Verification items for this drawing (mm, ordinates from the low corner). A direction names the side the tool comes from. Give positions to 0.01 mm unless a question says otherwise; leave off trailing zeros. Loops run counter-clockwise (first coordinate to the right, second up) from the corner with the lowest first, then second, coordinate; pieces in that order, holes last. Notation, with made-up numbers: M 3,38.25 L 58,38.25 A25 cw 58,74.25 Z; hole C 2,70 d1. An arc over 180 degrees is marked long. Use one line per item in the form item = value.
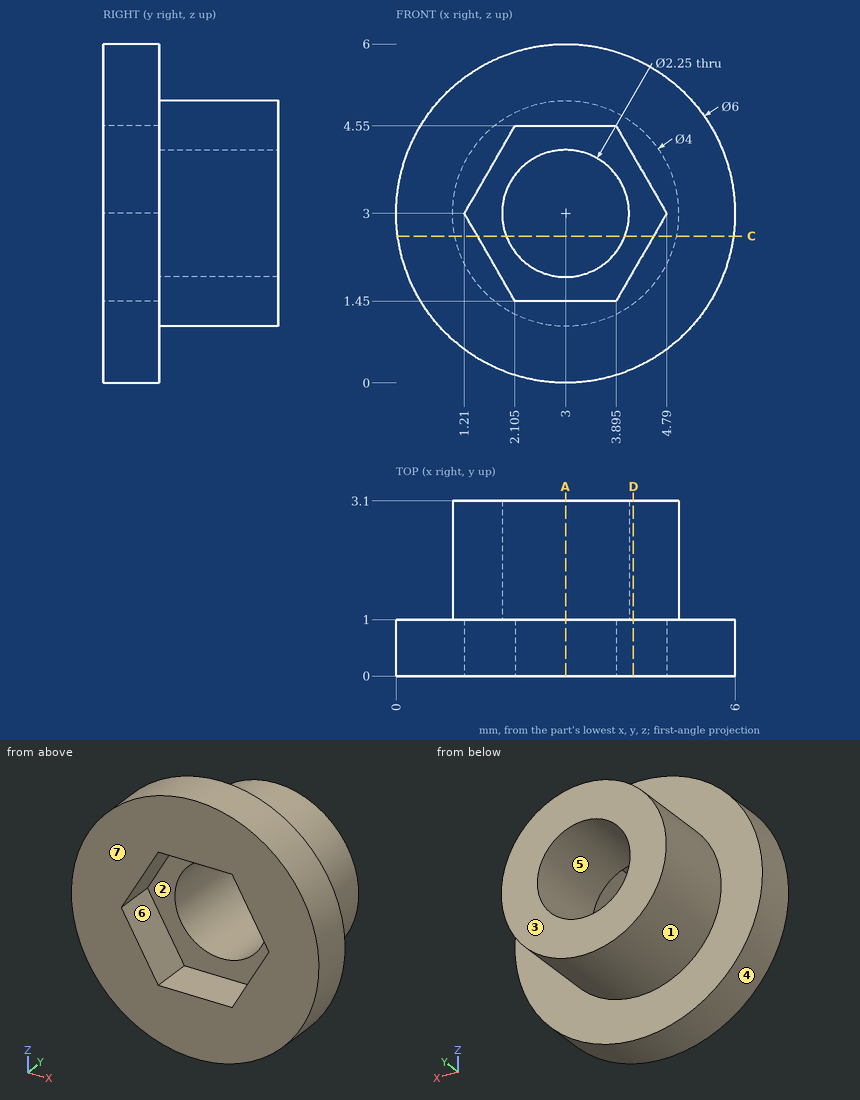
1) Section check A-A (x = 3). Record the cut outline in (y, z) (3 decimals).
Evaluation:
outline = M 0,0 L 1,0 L 1,1 L 3.1,1 L 3.1,1.875 L 1,1.875 L 1,1.45 L 0,1.45 Z; M 0,4.55 L 1,4.55 L 1,4.125 L 3.1,4.125 L 3.1,5 L 1,5 L 1,6 L 0,6 Z
2) Depth check by flat-ended pin: pin 1 Ø1 at (y, z) = (2, 3) entering from +X; pin 2 Ø1 at (x, y) = (1, 0.5) entering from -Z; pin 3 Ø1 at (x, z) = (2, 3) entering from -Y; pin 4 Ø2 at (x, z) = (3, 3) entering from +Y. Enter the tip coordinate at first touch or a pass-through.
Evaluation:
pin_1 = 5
pin_2 = 0.4
pin_3 = 1
pin_4 = through
3) Set-up check for the marked faces 1, 2 and 3: record each of +Z, -Z, +X, -X, +Y, -Y from which the full face is reachable in a straight line by a thin tool's end or side.
Evaluation:
face_1 = +Y
face_2 = -Y
face_3 = +Z, -Z, +X, -X, +Y
4) Scan lines: line 1 (X direction, y = 1.55, z = 3) (3 decimals); line 2 (Y direction, x = 5.45, z = 1.75); line 3 (Z direction, x = 3.6, y = 1.4). Record each from-to range of solid material in increasing order.
Evaluation:
line_1 = 1 to 1.875, 4.125 to 5
line_2 = 0 to 1
line_3 = 1.09 to 2.05, 3.95 to 4.91
5) Section check C-C (z = 2.6). Record the cut outline in (x, y).
Evaluation:
outline = M 0.03,0 L 1.44,0 L 1.44,1 L 1.95,1 L 1.95,3.1 L 1.04,3.1 L 1.04,1 L 0.03,1 Z; M 4.05,1 L 4.56,1 L 4.56,0 L 5.97,0 L 5.97,1 L 4.96,1 L 4.96,3.1 L 4.05,3.1 Z
6) Release check for a two-part mould opening along Z. For the marked faces 4, 5, 6 and 7 record: pulls with the +Z half, pulls with the -Z half, needs draft (parallel to the pull), parting line crosses it, or undercut.
Evaluation:
face_4 = parting line crosses it
face_5 = undercut
face_6 = undercut
face_7 = needs draft
7) Section check D-D (x = 4.2). Record the cut outline in (y, z), then the cut area to 3 significant figures.
Evaluation:
outline = M 0,0.25 L 1,0.25 L 1,1.4 L 3.1,1.4 L 3.1,4.6 L 1,4.6 L 1,5.75 L 0,5.75 L 0,4.02 L 1,4.02 L 1,1.98 L 0,1.98 Z
area = 10.2 mm^2
